Work out the finished part from the listing and answer in its coordinate system (mm). Face numbers are marked on the shaded views. A direction names the side the tool comes from. Give positions to 0.01 mm unless a question says otherwise; leave off trailing zeros. Loops run counter-clockwise (first coordinate to the right, second up) from the corner with the lowest first, then second, coordinate; pieces in that order, holes last.
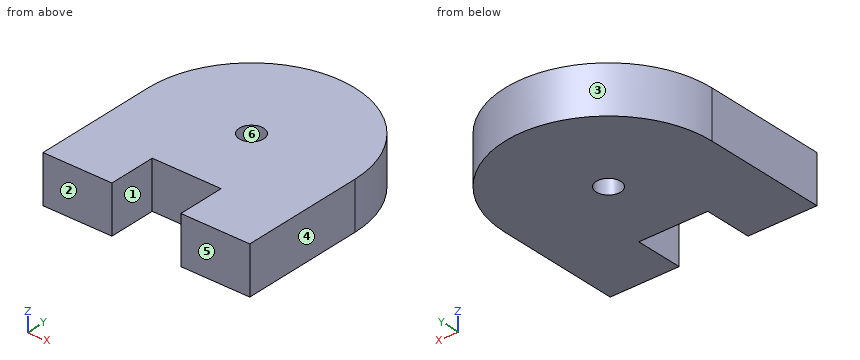
```python
from build123d import *

# Parameters (mm, degrees)
SKETCH1_R           = 1.5
BOSS_EXTRUDE1_DEPTH = 5.842
SKETCH3_W           = 8.466666667
SKETCH3_H           = 5.842
CUT_EXTRUDE2_DEPTH  = 5.842


with BuildPart() as part:
    # Sketch1 → Boss-Extrude1 (new body)
    with BuildSketch(Plane.XY):
        with BuildLine():
            Line((10.22047619, -9.525), (-15.17952381, -9.525))
            Line((-15.17952381, -9.525), (-15.17952381, 5.715))
            ThreePointArc((-15.17952381, 5.715), (-2.47952381, 18.415), (10.22047619, 5.715))
            Line((10.22047619, 5.715), (10.22047619, -9.525))
        make_face()
        with Locations((-2.47952381, 5.715)):
            Circle(SKETCH1_R, mode=Mode.SUBTRACT)
    extrude(amount=BOSS_EXTRUDE1_DEPTH)

    # Sketch3 → Cut-Extrude2 (cut)
    with BuildSketch(Plane.XY.offset(5.842)):
        with Locations((-2.47952381, -6.604)):
            Rectangle(SKETCH3_W, SKETCH3_H)
    extrude(amount=-CUT_EXTRUDE2_DEPTH, mode=Mode.SUBTRACT)


solid = part.part
```
Q1. Section C-C on x = -1.5 is taken. Give the vertices of the cut face in (y, z).
Q2. Determine the mould class of the marked faces 3, 4, 5 and 6 for opening direction Y: +Y half, -Y half, draft (parallel to the pull), parting line (faces both ways), or undercut.
Q3. Given pin 1 (3 mm diameter, centred on x = -4, z = 3, fed in from -Y), flat-ended and moving along its own axis, determine where the tip first touches the part or whether it passes through.
Q4. Section A-A on y = -6.5 is taken. Give the vertices of the cut face in (x, z).
Q5. Section B-B on z = 3.6 is taken. Give the vertices of the cut face in (x, y) (3 decimals).
Q6. Section D-D on x = 3.5 is taken. Give the vertices of the cut face in (y, z) (3 decimals).
Q7. Consider line 1 along X through (y, z) = (5.5, 3.3); line 2 along Y through (x, z) = (-2, 5.4); line 3 along Y through (x, z) = (-2.25, 5.3). Determine where each line is inside the solid, lowest interval first.
Q8. Which of the six approach directions +Z, -Z, +X, -X, +Y, -Y give full straight-line access (tool end or side, diameter ignored) to the marked faces 1 and 2?
Check result:
1. outline: (-3.68, 0) - (4.58, 0) - (4.58, 5.84) - (-3.68, 5.84) - close; (6.85, 0) - (18.38, 0) - (18.38, 5.84) - (6.85, 5.84) - close
2. face 3: +Y half
2. face 4: draft
2. face 5: -Y half
2. face 6: undercut
3. pin 1: stops at y = -3.68
4. outline: (-15.18, 0) - (-6.71, 0) - (-6.71, 5.84) - (-15.18, 5.84) - close; (1.75, 0) - (10.22, 0) - (10.22, 5.84) - (1.75, 5.84) - close
5. outline: (-15.18, -9.525) - (-6.713, -9.525) - (-6.713, -3.683) - (1.754, -3.683) - (1.754, -9.525) - (10.22, -9.525) - (10.22, 5.715) arc R12.7 ccw to (-15.18, 5.715) - close; hole circle Ø3 at (-2.48, 5.715)
6. outline: (-9.525, 0) - (16.919, 0) - (16.919, 5.842) - (-9.525, 5.842) - close
7. line 1: x = -15.18 to -3.96, -1 to 10.22
7. line 2: y = -3.68 to 4.29, 7.14 to 18.41
7. line 3: y = -3.68 to 4.23, 7.2 to 18.41
8. face 1: +Z, -Z, -Y
8. face 2: +Z, -Z, +X, -X, -Y
